Model file for the job. Use its own axes, mm. Give positions to 0.01 mm unless a question says otherwise; leave off trailing zeros. Write each loop counter-clockwise with the first axis right and the second up, starting at its lowest first coordinate (ties: lowest second). Pieces come first, ordered by that corner, then holes. Notation, with made-up numbers: (-30.5, 17.5) - (-22.5, 17.5) arc R31 cw to (-22.5, 53.5) - close; hole circle Ø10 at (7, 20.25). An arc over 180 degrees is marked (long way). Use a Markdown table: item, result. Add a question column.
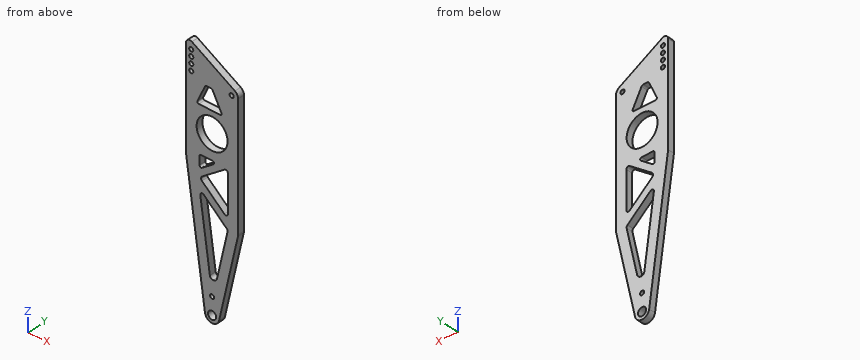
```python
from build123d import *

# Parameters (mm, degrees)
SKETCH1_R           = 3.96875
SKETCH1_R_2         = 15.08125
SKETCH1_R_3         = 2
BOSS_EXTRUDE1_DEPTH = 6.35
FILLET5_R           = 4.064
FILLET6_R           = 3.048
FILLET7_R           = 2.54
FILLET8_R           = 2.032
FILLET9_R           = 2.032
FILLET10_R          = 2.54
FILLET11_R          = 2.032
FILLET12_R          = 1.524
FILLET13_R          = 1.524
FILLET14_R          = 1.524
FILLET17_R          = 1.27
FILLET18_R          = 1.524
FILLET19_R          = 2.032
FILLET20_R          = 2.032


with BuildPart() as part:
    # Sketch1 → Boss-Extrude1 (new body)
    with BuildSketch(Plane(origin=(0, 0, 0), x_dir=(1, 0, 0), z_dir=(0, 1, 0))):
        with BuildLine():
            Line((25.4, -82.735721877), (25.4, -202.708825791))
            ThreePointArc((25.4, -202.708825791), (24.549261314, -205.883825791), (22.225, -208.208087105))
            Line((22.225, -208.208087105), (-19.685, -232.404836886))
            ThreePointArc((-19.685, -232.404836886), (-23.495, -232.404836886), (-25.4, -229.105280098))
            Line((-25.4, -229.105280098), (-25.4, -131.278691098))
            Line((-25.4, -131.278691098), (-6.917767735, 0.966806375))
            ThreePointArc((-6.917767735, 0.966806375), (-0.279220673, 6.97941694), (6.818426198, 1.51634072))
            Line((6.818426198, 1.51634072), (25.248569271, -81.357230313))
            ThreePointArc((25.248569271, -81.357230313), (25.362028789, -82.042329806), (25.4, -82.735721877))
        make_face()
        with Locations(Location((0, 0, 0), (0, 0, 270))):
            Circle(SKETCH1_R, mode=Mode.SUBTRACT)
        with Locations(Location((0, -160.246508934, 0), (0, 0, 270))):
            Circle(SKETCH1_R_2, mode=Mode.SUBTRACT)
        with Locations(Location((-20.32, -225.425, 0), (0, 0, 270))):
            Circle(SKETCH1_R_3, mode=Mode.SUBTRACT)
        with Locations(Location((-20.32, -219.075, 0), (0, 0, 270))):
            Circle(SKETCH1_R_3, mode=Mode.SUBTRACT)
        with Locations(Location((-20.32, -212.725, 0), (0, 0, 270))):
            Circle(SKETCH1_R_3, mode=Mode.SUBTRACT)
        with Locations(Location((-20.32, -206.375, 0), (0, 0, 270))):
            Circle(SKETCH1_R_3, mode=Mode.SUBTRACT)
        with Locations(Location((0, -16.51, 0), (0, 0, 270))):
            Circle(SKETCH1_R_3, mode=Mode.SUBTRACT)
        with Locations(Location((19.05, -202.708825791, 0), (0, 0, 270))):
            Circle(SKETCH1_R_3, mode=Mode.SUBTRACT)
        Polygon((4.14169212, -31.481995576), (15.384809867, -82.038158574), (-12.257886656, -106.330908852), (-1.797228059, -31.481995576), (0, -31.481995576), align=None, mode=Mode.SUBTRACT)
        Polygon((15.384809867, -91.891539471), (-12.257886656, -116.184289749), (15.384809867, -136.541766952), align=None, mode=Mode.SUBTRACT)
        Polygon((-12.257886656, -123.848026735), (4.97849313, -136.541766952), (-12.257886656, -136.541766952), align=None, mode=Mode.SUBTRACT)
        Polygon((-15.24, -180.566508934), (10.16, -180.566508934), (0, -199.967922148), (-6.35, -199.967922148), align=None, mode=Mode.SUBTRACT)
    extrude(amount=-BOSS_EXTRUDE1_DEPTH)

    # Fillet5
    fillet5_edges = [part.edges().sort_by_distance(p)[0] for p in [
        (4.14169212, -3.175, 31.481995576),
    ]]
    fillet(fillet5_edges, radius=FILLET5_R)

    # Fillet6
    fillet6_edges = [part.edges().sort_by_distance(p)[0] for p in [
        (-1.797228059, -3.175, 31.481995576),
    ]]
    fillet(fillet6_edges, radius=FILLET6_R)

    # Fillet7
    fillet7_edges = [part.edges().sort_by_distance(p)[0] for p in [
        (15.384809867, -3.175, 82.038158574),
    ]]
    fillet(fillet7_edges, radius=FILLET7_R)

    # Fillet8
    fillet8_edges = [part.edges().sort_by_distance(p)[0] for p in [
        (-12.257886656, -3.175, 106.330908852),
    ]]
    fillet(fillet8_edges, radius=FILLET8_R)

    # Fillet9
    fillet9_edges = [part.edges().sort_by_distance(p)[0] for p in [
        (15.384809867, -3.175, 91.891539471),
    ]]
    fillet(fillet9_edges, radius=FILLET9_R)

    # Fillet10
    fillet10_edges = [part.edges().sort_by_distance(p)[0] for p in [
        (-12.257886656, -3.175, 116.184289749),
    ]]
    fillet(fillet10_edges, radius=FILLET10_R)

    # Fillet11
    fillet11_edges = [part.edges().sort_by_distance(p)[0] for p in [
        (15.384809867, -3.175, 136.541766952),
    ]]
    fillet(fillet11_edges, radius=FILLET11_R)

    # Fillet12
    fillet12_edges = [part.edges().sort_by_distance(p)[0] for p in [
        (-12.257886656, -3.175, 123.848026735),
    ]]
    fillet(fillet12_edges, radius=FILLET12_R)

    # Fillet13
    fillet13_edges = [part.edges().sort_by_distance(p)[0] for p in [
        (4.97849313, -3.175, 136.541766952),
    ]]
    fillet(fillet13_edges, radius=FILLET13_R)

    # Fillet14
    fillet14_edges = [part.edges().sort_by_distance(p)[0] for p in [
        (-12.257886656, -3.175, 136.541766952),
    ]]
    fillet(fillet14_edges, radius=FILLET14_R)

    # Fillet17
    fillet17_edges = [part.edges().sort_by_distance(p)[0] for p in [
        (10.16, -3.175, 180.566508934),
    ]]
    fillet(fillet17_edges, radius=FILLET17_R)

    # Fillet18
    fillet18_edges = [part.edges().sort_by_distance(p)[0] for p in [
        (-15.24, -3.175, 180.566508934),
    ]]
    fillet(fillet18_edges, radius=FILLET18_R)

    # Fillet19
    fillet19_edges = [part.edges().sort_by_distance(p)[0] for p in [
        (-6.35, -3.175, 199.967922148),
    ]]
    fillet(fillet19_edges, radius=FILLET19_R)

    # Fillet20
    fillet20_edges = [part.edges().sort_by_distance(p)[0] for p in [
        (0, -3.175, 199.967922148),
    ]]
    fillet(fillet20_edges, radius=FILLET20_R)


solid = part.part
```
(1) Band-saw the part on A-A (z = 105.5). Write the cut outline in (x, y), then the cut area to 3 significant figures.
(2) Flat gauge pins, fed straight in: pin 1 (12 mm diameter, centred on x = 1.5, z = 170.5, fed in from +Y); pin 2 (3 mm diameter, centred on x = -4, y = -2.5, fed in from -Z); pin 3 (1.9 mm diameter, centred on x = -4, y = -2, fed in from +Z). Where does each tip first touch, or does it go through?
(3) Band-saw the part on C-C (y = -2.5). Give the number of separate pieces and of enclosed holes in the cut face, then the cut area to 3 significant figures.
(4) Band-saw the part on B-B (x = 19.05). Write the cut outline in (y, z).
(5) Probe probe 1 along X at (y, z) = (-2.75, 126); probe 2 along X at (y, z) = (-5.25, 160); probe 3 along Z at (x, y) = (4, -5). List the from-to ranges inside material, lowest first. Write a range as [from, to].
Model answer:
| question | item | result |
|---|---|---|
| 1 | outline | (-21.8, -6.35) - (-0.1, -6.35) - (-0.1, 0) - (-21.8, 0) - close; (15.38, -6.35) - (25.4, -6.35) - (25.4, 0) - (15.38, 0) - close |
| 1 | area | 201 mm^2 |
| 2 | pin 1 | stops at y = 0 |
| 2 | pin 2 | stops at z = -6.52 |
| 2 | pin 3 | stops at z = 223.9 |
| 3 | separate pieces | 1 |
| 3 | enclosed holes | 12 |
| 3 | area | 6,440 mm^2 |
| 4 | outline | (-6.35, 53.48) - (0, 53.48) - (0, 200.71) - (-6.35, 200.71) - close; (-6.35, 204.71) - (0, 204.71) - (0, 210.04) - (-6.35, 210.04) - close |
| 5 | probe 1 | x = [-24.66, -11.99], [-9.34, 1.07], [15.38, 25.4] |
| 5 | probe 2 | x = [-25.4, -15.08], [15.08, 25.4] |
| 5 | probe 3 | z = [-5.73, 32.94], [92.04, 101.9], [128.16, 145.71], [174.79, 180.57], [192.33, 218.73] |
